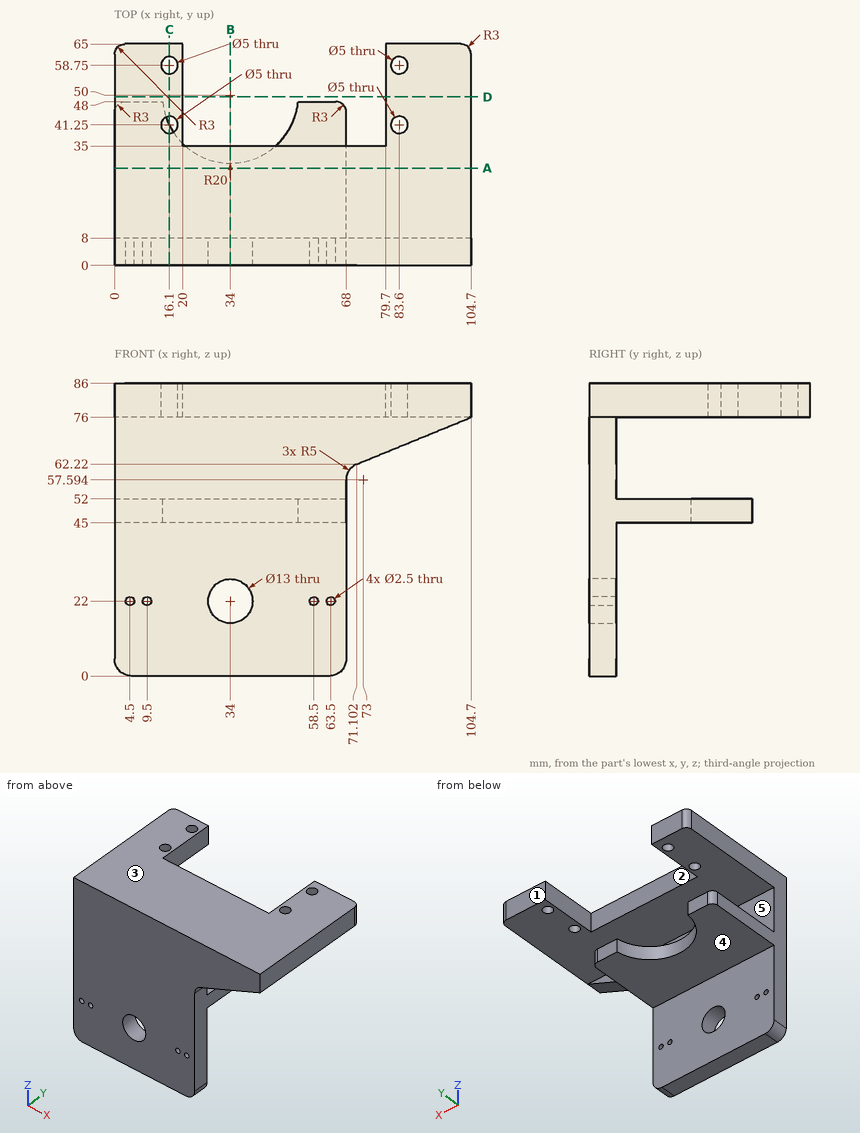
Here's the drawing with two shaded views (mm, measured from the low corner). I have some questions. A direction names the side the tool comes from. Give positions to 0.01 mm unless a question says otherwise; leave off trailing zeros. Loops run counter-clockwise (first coordinate to the right, second up) from the corner with the lowest first, then second, coordinate; pieces in that order, holes last. Notation, with made-up numbers: M -20,84.5 L 34,84.5 A16 cw 34,104.5 Z; hole C -9.5,55 d5. An arc over 180 degrees is marked long. Use one line per item in the form item = value. Start each with the question number.
(1) I want a section at C-C, the plane x = 16.1. Write out the boundary of the cut face in (y, z).
(2) I'm going to push flat-ended pins straight in: P1, Ø7.5, axis at x = 61, z = 49.5, coming from the +Y side; P2, Ø4, axis at x = 83.6, y = 58.75, coming from the +Z side; P3, Ø1, axis at x = 15, z = 38.5, coming from the +Y side; P4, Ø3, axis at x = 84.5, y = 37, coming from the -Z side. Where does each tip first touch, or does it pass through?
(3) Thinking about a two-plate mould opening in X: for the marked faces 1 and 2, which applies, released by +X, released by -X, zero draft, split by the parting line, or undercut?
(4) I want a section at D-D, the plane y = 49.5. Write out the boundary of the cut face in (x, z), and give its area (3 significant figures).
(5) On a 3-axis mill with a long thin cutter (end or side, diameter ignored), from which of +Z, -Z, +X, -X, +Y, -Y can I reach the whole of each face in a straight line? I mean the marked faces 3, 4 and 5. Say none if no direction works.
(6) Please list where these lines run through material, in increasing order: line 1 (Y direction, x = 16.1, z = 81.5); line 2 (X direction, y = 3.25, z = 22); line 3 (Z direction, x = 55, y = 24.5).
(7) I want a section at A-A, the plane y = 28.5. Write out the boundary of the cut face in (x, z), and give its area (3 significant figures).
(8) I want a section at B-B, the plane x = 34. Write out the boundary of the cut face in (y, z).
Worked out:
q1.outline = M 0,0 L 8,0 L 8,45 L 41.08,45 L 41.08,52 L 8,52 L 8,76 L 38.75,76 L 38.75,86 L 0,86 Z; M 43.75,76 L 56.25,76 L 56.25,86 L 43.75,86 Z; M 61.25,76 L 65,76 L 65,86 L 61.25,86 Z
q2.P1 = 48
q2.P2 = through
q2.P3 = 8
q2.P4 = 76
q3.face_1 = zero draft
q3.face_2 = undercut
q4.outline = M 0,76 L 20,76 L 20,86 L 0,86 Z; M 79.7,76 L 104.7,76 L 104.7,86 L 79.7,86 Z
q4.area = 450 mm²
q5.face_3 = +Z, +X, -X, +Y, -Y
q5.face_4 = -Z, +X, -X, +Y
q5.face_5 = +X, -X, +Y
q6.line_1 = 0 to 38.75, 43.75 to 56.25, 61.25 to 65
q6.line_2 = 0 to 3.25, 5.75 to 8.25, 10.75 to 27.5, 40.5 to 57.25, 59.75 to 62.25, 64.75 to 68
q6.line_3 = 45 to 52, 76 to 86
q7.outline = M 0,45 L 68,45 L 68,52 L 0,52 Z; M 0,76 L 104.7,76 L 104.7,86 L 0,86 Z
q7.area = 1,520 mm²
q8.outline = M 0,0 L 8,0 L 8,15.5 L 0,15.5 Z; M 0,28.5 L 8,28.5 L 8,45 L 30,45 L 30,52 L 8,52 L 8,76 L 35,76 L 35,86 L 0,86 Z
